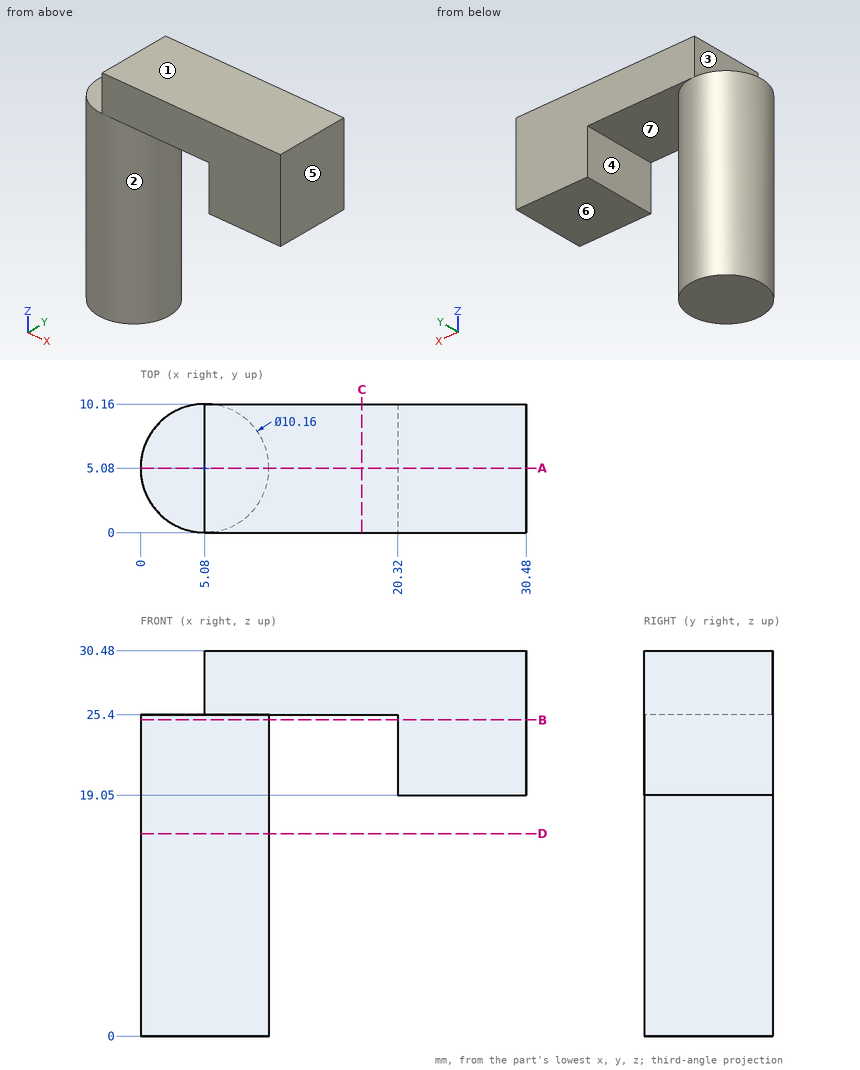
Here's the drawing with two shaded views (mm, measured from the low corner). I have some questions. A direction names the side the tool comes from. Round coordinates to 2 decimals unless told otherwise and drop trailing zeros. Write each loop counter-clockwise with the first axis right and the second up, starting at its lowest first coordinate (ties: lowest second). Pieces come first, ordered by that corner, then holes. Notation, with made-up numbers: M 13.5,73.25 L 45.5,73.25 A22 ccw 45.5,101.25 Z; hole C 23.5,53 d9. An arc over 180 degrees is marked long. Answer in a Markdown table with one row per item. Add a question column.
Q1. Imagine slicing it at C-C (x = 17.5). Please give me the cut outline in (y, z), then the cut area to 3 significant figures.
Q2. Imagine slicing it at D-D (z = 16). Please give me the cut outline in (x, y).
Q3. Imagine slicing it at B-B (z = 25). Please give me the cut outline in (x, y).
Q4. Will these pins go through, and if not, where does the flat tip stop? pin 1 Ø1.5 at (y, z) = (5, 27.5) entering from -X; pin 2 Ø6 at (x, y) = (17, 3.5) entering from -Z; pin 3 Ø1.5 at (x, z) = (12, 8) entering from +Y; pin 4 Ø5 at (x, y) = (23.5, 4) entering from -Z.
Q5. On a 3-axis mill with a long thin cutter (end or side, diameter ignored), from which of +Z, -Z, +X, -X, +Y, -Y can I reach the whole of each face in a straight line? I mean the marked faces 1, 2, 3 and 4. Say none if no direction works.
Q6. Imagine slicing it at A-A (y = 5.08). Please give me the cut outline in (x, z), then the cut area to 3 significant figures.
Q7. If I drill on line 1 (Z direction, x = 14.5, y = 6.25); line 2 (X direction, y = 1.75, z = 26.5); line 3 (X direction, y = 8.25, z = 19.5), over which ranges is the centre line in solid material (lowest first)? Write a range as from..to.
Q8. If we mould it in two halves opening along X, with no side actions, what happens to the marked faces 5, 6 and 7? For each: +X half, -X half, draft (parallel to the pull), parting line (faces both ways), or undercut.
Values:
| question | item | result |
|---|---|---|
| 1 | outline | M 0,25.4 L 10.16,25.4 L 10.16,30.48 L 0,30.48 Z |
| 1 | area | 51.6 mm^2 |
| 2 | outline | C 5.08,5.08 d10.16 |
| 3 | outline | C 5.08,5.08 d10.16; M 20.32,0 L 30.48,0 L 30.48,10.16 L 20.32,10.16 Z |
| 4 | pin 1 | x = 5.08 |
| 4 | pin 2 | z = 25.4 |
| 4 | pin 3 | through |
| 4 | pin 4 | z = 19.05 |
| 5 | face 1 | +Z, +X, -X, +Y, -Y |
| 5 | face 2 | -Z |
| 5 | face 3 | +Z, -X, +Y, -Y |
| 5 | face 4 | -Z, +Y, -Y |
| 6 | outline | M 0,0 L 10.16,0 L 10.16,25.4 L 20.32,25.4 L 20.32,19.05 L 30.48,19.05 L 30.48,30.48 L 5.08,30.48 L 5.08,25.4 L 0,25.4 Z |
| 6 | area | 452 mm^2 |
| 7 | line 1 | 25.4..30.48 |
| 7 | line 2 | 5.08..30.48 |
| 7 | line 3 | 1.11..9.05, 20.32..30.48 |
| 8 | face 5 | +X half |
| 8 | face 6 | draft |
| 8 | face 7 | undercut |
